from build123d import *

# Parameters (mm, degrees)
ESQUISSE1_W                  = 20
ESQUISSE1_H                  = 20
BOSS_EXTRU_1_DEPTH           = 10
ENL_V_MAT_EXTRU_1_DEPTH      = 11
ESQUISSE4_R                  = 2
ENL_V_MAT_EXTRU_2_DEPTH      = 142.139610307
ENL_V_MAT_EXTRU_2_DEPTH_BACK = 137.139610307
ENL_V_MAT_EXTRU_3_DEPTH      = 11.0000001
ENL_V_MAT_EXTRU_4_DEPTH      = 11
ENL_V_MAT_EXTRU_5_DEPTH      = 2
ESQUISSE9_R                  = 2.5
ENL_V_MAT_EXTRU_6_DEPTH      = 11


with BuildPart() as part:
    # Esquisse1 → Boss.-Extru.1 (new body)
    with BuildSketch(Plane(origin=(0, 0, 0), x_dir=(1, 0, 0), z_dir=(0, 1, 0))):
        with BuildLine():
            Line((-28.284271247, 28.284271247), (70.710678119, 141.421356237))
            ThreePointArc((70.710678119, 141.421356237), (141.421356237, 141.421356237), (141.421356237, 70.710678119))
            Line((141.421356237, 70.710678119), (28.284271247, -28.284271247))
            ThreePointArc((28.284271247, -28.284271247), (-28.284271247, -28.284271247), (-28.284271247, 28.284271247))
        make_face()
        Rectangle(ESQUISSE1_W, ESQUISSE1_H, mode=Mode.SUBTRACT)
    extrude(amount=BOSS_EXTRU_1_DEPTH)

    # Esquisse3 → Enlèv. mat.-Extru.1 (cut, through all)
    with BuildSketch(Plane(origin=(0, 10, 0), x_dir=(1, 0, 0), z_dir=(0, 1, 0))):
        Polygon((-8.232233047, -11.767766953), (-27.234385984, -30.76991989), (-30.76991989, -27.234385984), (-11.767766953, -8.232233047), (-9.726873799, -6.191339893), (-6.191339893, -9.726873799), align=None)
    extrude(amount=-ENL_V_MAT_EXTRU_1_DEPTH, mode=Mode.SUBTRACT)

    # Esquisse4 → Enlèv. mat.-Extru.2 (cut, two sides)
    with BuildSketch(Plane(origin=(1.767766953, 0, 1.767766953), x_dir=(-0.707106781, 0, 0.707106781), z_dir=(-0.707106781, 0, -0.707106781))) as enl_v_mat_extru_2_sk:
        with Locations((35.022819071, 6)):
            Circle(ESQUISSE4_R)
    extrude(amount=ENL_V_MAT_EXTRU_2_DEPTH, mode=Mode.SUBTRACT)
    extrude(enl_v_mat_extru_2_sk.sketch, amount=-ENL_V_MAT_EXTRU_2_DEPTH_BACK, mode=Mode.SUBTRACT)

    # Esquisse5 → Enlèv. mat.-Extru.3 (cut, through all)
    with BuildSketch(Plane(origin=(0, 10, 0), x_dir=(1, 0, 0), z_dir=(0, 1, 0))):
        Polygon((-34.683660608, -14.703220533), (-36.451427561, -16.470987486), (-40.908486709, -7.777625617), (-39.491104164, -6.360243072), (-32.915893655, -12.93545358), align=None)
        Polygon((-7.777625617, -40.908486709), (-6.360243072, -39.491104164), (-12.93545358, -32.915893655), (-14.703220533, -34.683660608), (-16.470987486, -36.451427561), align=None)
    extrude(amount=-ENL_V_MAT_EXTRU_3_DEPTH, mode=Mode.SUBTRACT)

    # Esquisse7 → Enlèv. mat.-Extru.4 (cut, through all)
    with BuildSketch(Plane(origin=(0, 10, 0), x_dir=(1, 0, 0), z_dir=(0, 1, 0))):
        with BuildLine():
            Line((91.923881554, 98.994949366), (102.530483272, 109.601551084))
            ThreePointArc((102.530483272, 109.601551084), (109.601551084, 109.601551084), (109.601551084, 102.530483272))
            Line((109.601551084, 102.530483272), (98.994949366, 91.923881554))
            ThreePointArc((98.994949366, 91.923881554), (91.923881554, 91.923881554), (91.923881554, 98.994949366))
        make_face()
        with BuildLine():
            Line((94.045201898, 119.373629023), (104.651803616, 129.98023074))
            ThreePointArc((104.651803616, 129.98023074), (107.48023074, 129.98023074), (107.48023074, 127.151803616))
            Line((107.48023074, 127.151803616), (96.873629023, 116.545201898))
            ThreePointArc((96.873629023, 116.545201898), (94.045201898, 116.545201898), (94.045201898, 119.373629023))
        make_face()
        with BuildLine():
            Line((71.545201898, 96.873629023), (82.151803616, 107.48023074))
            ThreePointArc((82.151803616, 107.48023074), (84.98023074, 107.48023074), (84.98023074, 104.651803616))
            Line((84.98023074, 104.651803616), (74.373629023, 94.045201898))
            ThreePointArc((74.373629023, 94.045201898), (71.545201898, 94.045201898), (71.545201898, 96.873629023))
        make_face()
        with BuildLine():
            Line((119.373629023, 94.045201898), (129.98023074, 104.651803616))
            ThreePointArc((129.98023074, 104.651803616), (129.98023074, 107.48023074), (127.151803616, 107.48023074))
            Line((127.151803616, 107.48023074), (116.545201898, 96.873629023))
            ThreePointArc((116.545201898, 96.873629023), (116.545201898, 94.045201898), (119.373629023, 94.045201898))
        make_face()
        with BuildLine():
            Line((96.873629023, 71.545201898), (107.48023074, 82.151803616))
            ThreePointArc((107.48023074, 82.151803616), (107.48023074, 84.98023074), (104.651803616, 84.98023074))
            Line((104.651803616, 84.98023074), (94.045201898, 74.373629023))
            ThreePointArc((94.045201898, 74.373629023), (94.045201898, 71.545201898), (96.873629023, 71.545201898))
        make_face()
    extrude(amount=-ENL_V_MAT_EXTRU_4_DEPTH, mode=Mode.SUBTRACT)

    # Esquisse8 → Enlèv. mat.-Extru.5 (cut)
    with BuildSketch(Plane(origin=(0, 10, 0), x_dir=(1, 0, 0), z_dir=(0, 1, 0))):
        with BuildLine():
            Line((123.743686708, 88.388347648), (113.13708499, 77.781745931))
            ThreePointArc((113.13708499, 77.781745931), (77.781745931, 77.781745931), (77.781745931, 113.13708499))
            Line((77.781745931, 113.13708499), (88.388347648, 123.743686708))
            ThreePointArc((88.388347648, 123.743686708), (123.743686708, 123.743686708), (123.743686708, 88.388347648))
        make_face()
    extrude(amount=-ENL_V_MAT_EXTRU_5_DEPTH, mode=Mode.SUBTRACT)

    # Esquisse9 → Enlèv. mat.-Extru.6 (cut, through all)
    with BuildSketch(Plane(origin=(0, 0, 0), x_dir=(-1, 0, 0), z_dir=(0, -1, 0))):
        with Locations((-70.710678119, 141.421356237)):
            Circle(ESQUISSE9_R)
        with Locations((-98.244293926, 155.450434208)):
            Circle(ESQUISSE9_R)
        with Locations((-128.765542165, 150.616343387)):
            Circle(ESQUISSE9_R)
        with Locations((-150.616343387, 128.765542165)):
            Circle(ESQUISSE9_R)
        with Locations((-155.450434208, 98.244293926)):
            Circle(ESQUISSE9_R)
        with Locations((-141.421356237, 70.710678119)):
            Circle(ESQUISSE9_R)
        with Locations((-115.287543419, 47.843591903)):
            Circle(ESQUISSE9_R)
    extrude(amount=-ENL_V_MAT_EXTRU_6_DEPTH, mode=Mode.SUBTRACT)


solid = part.part
Read the model definition and answer for the solid it produces. Units are mm, in the model's axes. A direction names the side the tool comes from. Round coordinates to 2 decimals unless told otherwise and drop trailing zeros. Write each loop counter-clockwise with the first axis right and the second up, starting at its lowest first coordinate (ties: lowest second). Pieces come first, ordered by that corner, then holes.
1. The part is cut by section A-A, the plane x = -2. Determine the outline of the cut face in (y, z).
2. The part is cut by section B-B, the plane y = 2. State how many separate pieces and enclosed holes the cut face has, then the cut area to 3 significant figures.
3. The part is cut by section C-C, the plane z = -19.5. Determine the outline of the cut face in (x, y).
4. Which of the six approach directions +Z, -Z, +X, -X, +Y, -Y give full straight-line access (tool end or side, diameter ignored) to faces 3 (the face through (102.25, 4.06, -121.92)), 4 (the face through (-33.55, 4.93, 21.78)), 5 (the face through (128.511, 4.93, -59.414)), 6 (the face through (-36.25, 5.07, 9.6)), 7 (the face through (123.35, 9.01, -124.13))?
5. Given pin 1 Ø1 at (y, z) = (6, -89) entering from +X; pin 2 Ø1 at (x, z) = (76, -80.5) entering from -Y; pin 3 Ø5 at (x, y) = (-5, 4.5) entering from +Z; pin 4 Ø4 at (x, y) = (35.5, 8) entering from +Z, each flat-ended and moving along its own axis, determine where each tip first touches the part or whether it passes through.
6. Straight lines are drawn through the part: L1, parallel to X at y = 5.5, z = -101.5; L2, parallel to Z at x = 104, y = 5.75; L3, parallel to Z at x = 98.5, y = 3.5. For each, find the intervals that lie inside material, in ascending order.
7. The part is cut by section D-D, the plane x = 44.5. Determine the outline of the cut face in (y, z).
8. Determine the mould class of faces 1 (the face through (78.17, 9.01, -77.4)), 2 (the face through (-20.25, 5.23, 31.89)) for opening direction Y: pulls with the +Y half, pulls with the -Y half, needs draft (parallel to the pull), parting line crosses it, or undercut.
Values:
1. outline: (0, -58.32) - (10, -58.32) - (10, -10) - (0, -10) - close; (0, 10) - (10, 10) - (10, 39.95) - (0, 39.95) - close
2. separate pieces: 1
2. enclosed holes: 5
2. area: 18,800 mm2
3. outline: (-34.92, 0) - (82.89, 0) - (82.89, 10) - (-34.92, 10) - close
4. face 3: +Y, -Y
4. face 4: +Z, -X, +Y, -Y
4. face 5: +Z, +X, +Y, -Y
4. face 6: -X, +Y, -Y
4. face 7: +Y
5. pin 1: stops at x = 153.24
5. pin 2: stops at y = 0
5. pin 3: stops at z = 39.92
5. pin 4: stops at z = 23.72
6. L1: x = 35.78 to 76.17, 81.83 to 94.43, 108.57 to 121.17, 126.83 to 155.86
6. L2: z = -156.02 to -129.33, -123.67 to -110.62, -96.93 to -84.33, -78.67 to -37.97
6. L3: z = -152.96 to -123.83, -118.17 to -105.57, -91.49 to -78.83, -73.17 to -33.15
7. outline: (0, -111.47) - (10, -111.47) - (10, 14.1) - (0, 14.1) - close
8. face 1: needs draft
8. face 2: undercut
